Build history of the part. All positions in model axes, mm. Face numbers are marked on the shaded views. A direction names the side the tool comes from. Round coordinates to 2 decimals unless told otherwise and drop trailing zeros. Write each loop counter-clockwise with the first axis right and the second up, starting at its lowest first coordinate (ties: lowest second). Pieces come first, ordered by that corner, then holes. Notation, with made-up numbers: M -18.75,-19 L 1.25,-19 A8 ccw 1.25,-6 Z; hole C -25,10 d8. An arc over 180 degrees is marked long. Write item = value, one per line. Start each with the question number.
Q1. Band-saw the part on C-C on x = -3.5. Write the cut outline in (y, z), plus the area to 3 significant figures.
Q2. Drop flat-ended pins along their axis: P1, Ø4, axis at x = -1, z = 14, coming from the -Y side; P2, Ø3, axis at x = 3, z = 11, coming from the +Y side; P3, Ø4, axis at y = 11, z = 3, coming from the +X side. Give the stop position or say it passes through.
Q3. Probe L1, parallel to Y at x = -3.85, z = 15; L2, parallel to X at y = 8, z = 12.25; L3, parallel to Y at x = -0.75, z = 2.5. List the from-to ranges inside material, lowest first.
Q4. Band-saw the part on B-B on y = 0. Write the cut outline in (x, z).
Q5. Pull direction X, two halves, no side cores. Call the marked faces 5, 6, 7 and 8: released by +X, released by -X, zero draft, split by the parting line, or undercut.
Q6. Band-saw the part on A-A on z = 9.75. Write the cut outline in (x, y).
Q7. Band-saw the part on D-D on y = -12.5. Write the cut outline in (x, z) (3 decimals).
Q8. Tool access for the marked faces 1, 2, 3 and 4: list every direction of +Z, -Z, +X, -X, +Y, -Y with a clear straight run to the whole face (end or side of a thin tool).
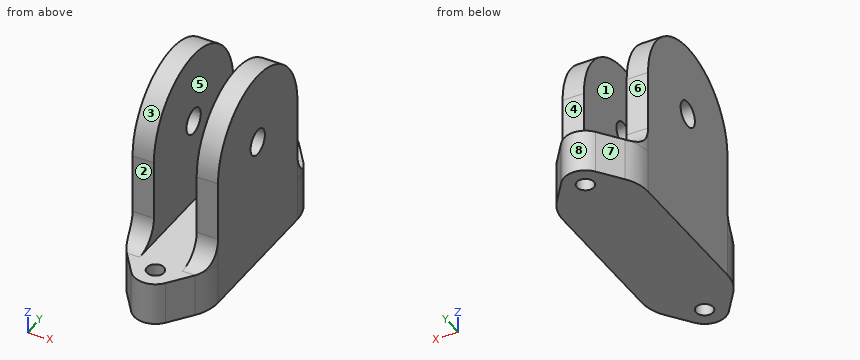
```python
from build123d import *

# Parameters (mm, degrees)
ESQUISSE1_R        = 1
BOSS_EXTRU_1_DEPTH = 5
ESQUISSE2_R        = 1.5
BOSS_EXTRU_2_DEPTH = 2.5
CONG_1_R           = 3


with BuildPart() as part:
    # Esquisse1 → Boss.-Extru.1 (new body)
    with BuildSketch(Plane.XY):
        with BuildLine():
            Line((-4, 11.333333333), (-2, 14))
            ThreePointArc((-2, 14), (0, 15), (2, 14))
            Line((2, 14), (4, 11.333333333))
            ThreePointArc((4, 11.333333333), (4.74341649, 9.914472163), (5, 8.333333333))
            Line((5, 8.333333333), (5, -8.333333333))
            ThreePointArc((5, -8.333333333), (4.74341649, -9.914472163), (4, -11.333333333))
            Line((4, -11.333333333), (2, -14))
            ThreePointArc((2, -14), (0, -15), (-2, -14))
            Line((-2, -14), (-4, -11.333333333))
            ThreePointArc((-4, -11.333333333), (-4.74341649, -9.914472163), (-5, -8.333333333))
            Line((-5, -8.333333333), (-5, 8.333333333))
            ThreePointArc((-5, 8.333333333), (-4.74341649, 9.914472163), (-4, 11.333333333))
        make_face()
        with Locations((0, 12.5)):
            Circle(ESQUISSE1_R, mode=Mode.SUBTRACT)
        with Locations((0, -12.5)):
            Circle(ESQUISSE1_R, mode=Mode.SUBTRACT)
    extrude(amount=BOSS_EXTRU_1_DEPTH)

    # Esquisse2 → Boss.-Extru.2 (add)
    with BuildSketch(Plane.ZY.offset(5)):
        with BuildLine():
            Line((5, 8.333333333), (15, 8.333333333))
            ThreePointArc((15, 8.333333333), (23.333333333, 0), (15, -8.333333333))
            Line((15, -8.333333333), (5, -8.333333333))
            Line((5, -8.333333333), (5, 8.333333333))
        make_face()
        with Locations((15, 0)):
            Circle(ESQUISSE2_R, mode=Mode.SUBTRACT)
    boss_extru_2 = extrude(amount=-BOSS_EXTRU_2_DEPTH)

    # Symétrie1: Boss.-Extru.2 across plane
    add(boss_extru_2.mirror(Plane(origin=(0, 0, 0), x_dir=(0, 0, 1), z_dir=(1, 0, 0))))

    # Congé1
    # the kernel refuses this fillet: 3 mm, written as the material it adds along each edge
    with BuildSketch(Plane(origin=(12.5, 8.333333333, 5), x_dir=(0, 1, 0), z_dir=(-1, 0, 0))) as cong_1_piece_1_section:
        with BuildLine():
            CenterArc((CONG_1_R, -CONG_1_R), CONG_1_R, 90, 90)
            Line((0, -CONG_1_R), (0, 0))
            Line((0, 0), (CONG_1_R, 0))
        make_face()
    cong_1_piece_1 = extrude(amount=10, mode=Mode.PRIVATE)
    cong_1_piece_1 = cong_1_piece_1 & Plane(origin=(0, 8.333333333, 5.683499062), x_dir=(-1, 0, 0), z_dir=(0, 0, -1)) * Cylinder(5, 32, mode=Mode.PRIVATE)
    add(cong_1_piece_1)
    with BuildSketch(Plane(origin=(12.5, 8.333333333, 5), x_dir=(0, 1, 0), z_dir=(-1, 0, 0))) as cong_1_piece_2_section:
        with BuildLine():
            CenterArc((CONG_1_R, -CONG_1_R), CONG_1_R, 90, 90)
            Line((0, -CONG_1_R), (0, 0))
            Line((0, 0), (CONG_1_R, 0))
        make_face()
    cong_1_piece_2 = extrude(amount=17.5, mode=Mode.PRIVATE)
    cong_1_piece_2 = cong_1_piece_2 & Plane(origin=(0, 8.333333333, 5.683498856), x_dir=(-1, 0, 0), z_dir=(0, 0, -1)) * Cylinder(5, 47, mode=Mode.PRIVATE)
    cong_1_piece_2 = split(cong_1_piece_2, bisect_by=Plane(origin=(-2.5, 8.977430515, 5.683498856), z_dir=(-1, 0, 0)), keep=Keep.TOP, mode=Mode.PRIVATE)
    add(cong_1_piece_2)
    with BuildSketch(Plane(origin=(12.5, -8.333333333, 5), x_dir=(0, -1, 0), z_dir=(-1, 0, 0))) as cong_1_piece_3_section:
        with BuildLine():
            CenterArc((CONG_1_R, CONG_1_R), CONG_1_R, 180, 90)
            Line((0, CONG_1_R), (0, 0))
            Line((0, 0), (CONG_1_R, 0))
        make_face()
    cong_1_piece_3 = extrude(amount=10, mode=Mode.PRIVATE)
    cong_1_piece_3 = cong_1_piece_3 & Plane(origin=(0, -8.333333333, 5.683498856), x_dir=(-0.8000000000000032, -0.5999999999999958, 0), z_dir=(0, 0, -1)) * Cylinder(5, 32, mode=Mode.PRIVATE)
    add(cong_1_piece_3)
    with BuildSketch(Plane(origin=(12.5, -8.333333333, 5), x_dir=(0, -1, 0), z_dir=(-1, 0, 0))) as cong_1_piece_4_section:
        with BuildLine():
            CenterArc((CONG_1_R, CONG_1_R), CONG_1_R, 180, 90)
            Line((0, CONG_1_R), (0, 0))
            Line((0, 0), (CONG_1_R, 0))
        make_face()
    cong_1_piece_4 = extrude(amount=17.5, mode=Mode.PRIVATE)
    cong_1_piece_4 = cong_1_piece_4 & Plane(origin=(0, -8.333333333, 5.683499062), x_dir=(-0.8000000000000032, -0.5999999999999958, 0), z_dir=(0, 0, -1)) * Cylinder(5, 47, mode=Mode.PRIVATE)
    cong_1_piece_4 = split(cong_1_piece_4, bisect_by=Plane(origin=(-2.5, -8.97743132, 5.683499062), z_dir=(-1, 0, 0)), keep=Keep.TOP, mode=Mode.PRIVATE)
    add(cong_1_piece_4)
    with BuildSketch(Plane(origin=(-12.5, 8.333333333, 5), x_dir=(0, 1, 0), z_dir=(1, 0, 0))) as cong_1_piece_5_section:
        with BuildLine():
            CenterArc((CONG_1_R, CONG_1_R), CONG_1_R, 180, 90)
            Line((0, CONG_1_R), (0, 0))
            Line((0, 0), (CONG_1_R, 0))
        make_face()
    cong_1_piece_5 = extrude(amount=10, mode=Mode.PRIVATE)
    cong_1_piece_5 = cong_1_piece_5 & Plane(origin=(0, 8.333333333, 5.683498856), x_dir=(-1, 0, 0), z_dir=(0, 0, -1)) * Cylinder(5, 32, mode=Mode.PRIVATE)
    add(cong_1_piece_5)
    with BuildSketch(Plane(origin=(-12.5, 8.333333333, 5), x_dir=(0, 1, 0), z_dir=(1, 0, 0))) as cong_1_piece_6_section:
        with BuildLine():
            CenterArc((CONG_1_R, CONG_1_R), CONG_1_R, 180, 90)
            Line((0, CONG_1_R), (0, 0))
            Line((0, 0), (CONG_1_R, 0))
        make_face()
    cong_1_piece_6 = extrude(amount=17.5, mode=Mode.PRIVATE)
    cong_1_piece_6 = cong_1_piece_6 & Plane(origin=(0, 8.333333333, 5.683499062), x_dir=(-1, 0, 0), z_dir=(0, 0, -1)) * Cylinder(5, 47, mode=Mode.PRIVATE)
    cong_1_piece_6 = split(cong_1_piece_6, bisect_by=Plane(origin=(2.5, 8.97743132, 5.683499062), z_dir=(1, 0, 0)), keep=Keep.TOP, mode=Mode.PRIVATE)
    add(cong_1_piece_6)
    with BuildSketch(Plane(origin=(-12.5, -8.333333333, 5), x_dir=(0, -1, 0), z_dir=(1, 0, 0))) as cong_1_piece_7_section:
        with BuildLine():
            CenterArc((CONG_1_R, -CONG_1_R), CONG_1_R, 90, 90)
            Line((0, -CONG_1_R), (0, 0))
            Line((0, 0), (CONG_1_R, 0))
        make_face()
    cong_1_piece_7 = extrude(amount=10, mode=Mode.PRIVATE)
    cong_1_piece_7 = cong_1_piece_7 & Plane(origin=(0, -8.333333333, 5.683499062), x_dir=(-0.8000000000000032, -0.5999999999999958, 0), z_dir=(0, 0, -1)) * Cylinder(5, 32, mode=Mode.PRIVATE)
    add(cong_1_piece_7)
    with BuildSketch(Plane(origin=(-12.5, -8.333333333, 5), x_dir=(0, -1, 0), z_dir=(1, 0, 0))) as cong_1_piece_8_section:
        with BuildLine():
            CenterArc((CONG_1_R, -CONG_1_R), CONG_1_R, 90, 90)
            Line((0, -CONG_1_R), (0, 0))
            Line((0, 0), (CONG_1_R, 0))
        make_face()
    cong_1_piece_8 = extrude(amount=17.5, mode=Mode.PRIVATE)
    cong_1_piece_8 = cong_1_piece_8 & Plane(origin=(0, -8.333333333, 5.683498856), x_dir=(-0.8000000000000032, -0.5999999999999958, 0), z_dir=(0, 0, -1)) * Cylinder(5, 47, mode=Mode.PRIVATE)
    cong_1_piece_8 = split(cong_1_piece_8, bisect_by=Plane(origin=(2.5, -8.977430515, 5.683498856), z_dir=(1, 0, 0)), keep=Keep.TOP, mode=Mode.PRIVATE)
    add(cong_1_piece_8)


solid = part.part
```
Conclusion:
q1.outline = M -12,0 L 12,0 L 12,5 L 11.33,5 A3 cw 8.33,8 L 8.33,15 A8.33 ccw -8.33,15 L -8.33,8 A3 cw -11.33,5 L -12,5 Z; hole C 0,15 d3
q1.area = 393 mm^2
q2.P1 = -8.33
q2.P2 = 8.33
q2.P3 = 4.96
q3.L1 = -8.33 to -1.5, 1.5 to 8.33
q3.L2 = -5 to -2.5, 2.5 to 5
q3.L3 = -14.88 to -13.16, -11.84 to 11.84, 13.16 to 14.88
q4.outline = M -5,0 L 5,0 L 5,13.5 L 2.5,13.5 L 2.5,5 L -2.5,5 L -2.5,13.5 L -5,13.5 Z; M -5,16.5 L -2.5,16.5 L -2.5,23.33 L -5,23.33 Z; M 2.5,16.5 L 5,16.5 L 5,23.33 L 2.5,23.33 Z
q5.face_5 = undercut
q5.face_6 = zero draft
q5.face_7 = released by -X
q5.face_8 = split by the parting line
q6.outline = M -5,-8.33 L -2.5,-8.33 L -2.5,8.33 L -5,8.33 Z; M 2.5,-8.33 L 5,-8.33 L 5,8.33 L 2.5,8.33 Z
q7.outline = M -3.125,0 L -1,0 L -1,5 L -3.125,5 Z; M 1,0 L 3.125,0 L 3.125,5 L 1,5 Z
q8.face_1 = +Z, +Y, -Y
q8.face_2 = +Z, +X, -X, -Y
q8.face_3 = +Z, +X, -X
q8.face_4 = +Z, +X, -X, +Y
